Answer from the drawing. Dimensions are ordinates in mm from the lowest x, y and z of the part. Give positions to 0.01 mm unless a question says otherwise; leave off trailing zeros. Order: outer loops, then holes, each group sorted by start corner. A loop starts at its lowest first (then second) coordinate and runs counter-clockwise, first axis right, second up.
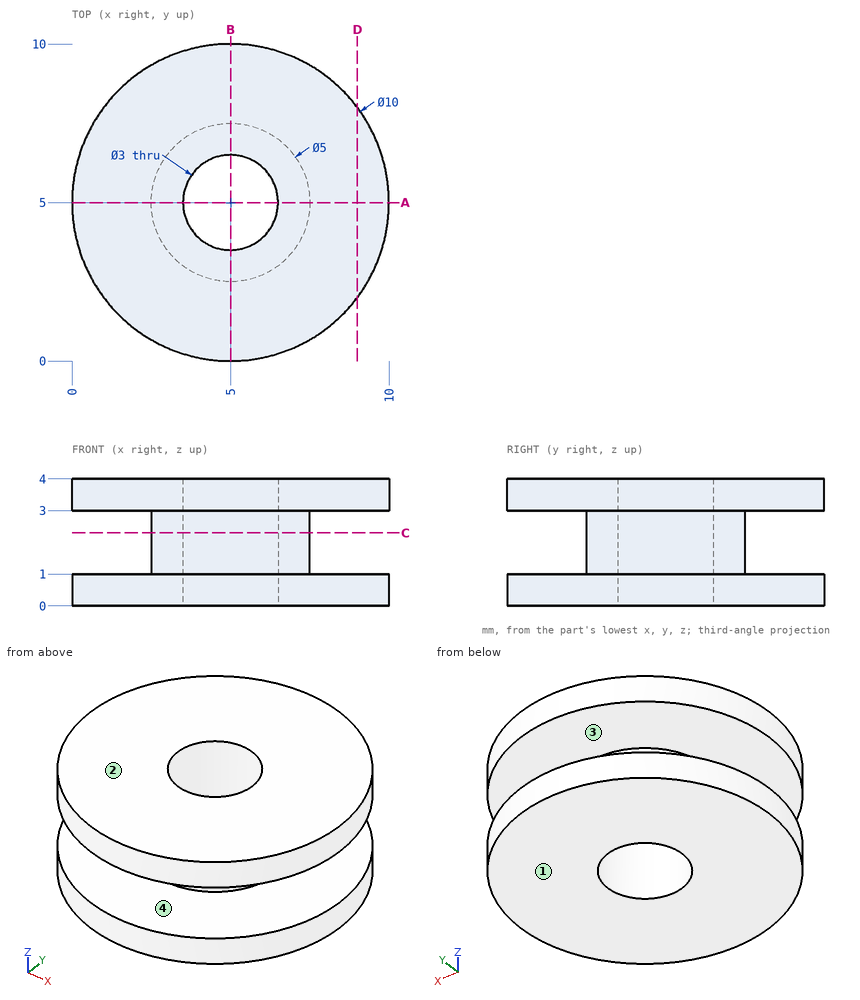
1) For a pull along Z with two mould halves and no side action, classify the marked faces 1, 2, 3 and 4 as released by +Z, released by -Z, zero draft, split by the parting line, or undercut.
Final values:
face 1: released by -Z
face 2: released by +Z
face 3: undercut
face 4: undercut
2) Consider L1, parallel to Y at x = 5, z = 2.7; L2, parallel to Z at x = 5.25, y = 1.25; L3, parallel to X at y = 7.5, z = 0.8. Determine where each line is inside the solid, lowest interval first.
Final values:
L1: y = 2.5 to 3.5, 6.5 to 7.5
L2: z = 0 to 1, 3 to 4
L3: x = 0.67 to 9.33
3) Given pin 1 (2 mm diameter, centred on x = 1.5, z = 1, fed in from -Y); pin 2 (1 mm diameter, centred on y = 2, z = 3, fed in from +X); pin 3 (1 mm diameter, centred on y = 2.5, z = 0.5, fed in from +X), each flat-ended and moving along its own axis, determine where each tip first touches the part or whether it passes through.
Final values:
pin 1: stops at y = 0.67
pin 2: stops at x = 9.33
pin 3: stops at x = 9.58
4) The part is cut by section C-C on z = 2.3. Determine the outline of the cut face in (x, y), and give its area (3 significant figures).
Final values:
outline: circle Ø5 at (5, 5); hole circle Ø3 at (5, 5)
area: 12.6 mm2
5) The part is cut by section A-A on y = 5. Determine the outline of the cut face in (x, z).
Final values:
outline: (0, 0) - (3.5, 0) - (3.5, 4) - (0, 4) - (0, 3) - (2.5, 3) - (2.5, 1) - (0, 1) - close; (6.5, 0) - (10, 0) - (10, 1) - (7.5, 1) - (7.5, 3) - (10, 3) - (10, 4) - (6.5, 4) - close
6) The part is cut by section D-D on x = 9. Determine the outline of the cut face in (y, z).
Final values:
outline: (2, 0) - (8, 0) - (8, 1) - (2, 1) - close; (2, 3) - (8, 3) - (8, 4) - (2, 4) - close
